Autodesk Inventor part; units mm, degrees
ref_plane "YZ Plane" through (0, 0, 0) normal (1, 0, 0) x (0, 1, 0)
ref_plane "XZ Plane" through (0, 0, 0) normal (0, 1, 0) x (-1, 0, 0)
ref_plane "XY Plane" through (0, 0, 0) normal (0, 0, 1) x (1, 0, 0)
sketch "Sketch1" plane through (0, 0, 0) normal (0, 0, 1) x (1, 0, 0)
  circle A0 centre (0, 0) radius 11
  dimension "d0" = 22
extrude "Extrusion1" add sketch "Sketch1" along normal mid plane 6
sketch "Sketch3" plane through (0, 0, 3) normal (0, 0, 1) x (1, 0, 0)
  point P0 (0, 0)
hole "Hole1" at (0, 0, 3) direction (0, 0, -1) diameter 10.376 end through all
sketch "Sketch2" plane through (0, 0, 3) normal (0, 0, 1) x (1, 0, 0)
  line L0 (11, 1) -> (10, 1)
  line L1 (10, 1) -> (10, -1)
  line L2 (10, -1) -> (11, -1)
  line L3 (11, -1) -> (11, 1)
  circle A0 centre (0, 0) radius 11 construction
  point P0 (10, 0)
  dimension "d3" = 2
  dimension "d4" = 1
extrude "Extrusion2" cut sketch "Sketch2" against normal through all
pattern_circular "Circular Pattern1" count 4 over 360 about axis through (0, 0, 0) along (0, 0, 1) of "Extrusion2"
chamfer "Chamfer1" distance 1 angle 45 4 edges at (7.7782, -7.7782, 3) (7.7782, 7.7782, 3) (-7.7782, 7.7782, 3) (-7.7782, -7.7782, 3)
properties material "Stainless Steel"
Read the model definition and answer for the solid it produces. Units are mm, in the model's axes. A direction names the side the tool comes from. Give positions to 0.01 mm unless a question says otherwise; leave off trailing zeros. Loops run counter-clockwise (first coordinate to the right, second up) from the corner with the lowest first, then second, coordinate; pieces in that order, holes last.
Item 1: For faces 1 (the flat face through (1, -10.5, 0)), 2 (the flat face through (-10.5, 1, 0)), 3 (the flat face through (0, 10, 0)), 4 (the flat face through (10.5, 1, 0)), determine the directions among +Z, -Z, +X, -X, +Y, -Y from which every point of the face is accessible in a straight line to the end or side of a thin tool.
Item 2: Each of these flat-tipped pins is pushed along its axis until it touches: pin 1 Ø1 at (x, z) = (2, 0) entering from +Y; pin 2 Ø1.6 at (x, z) = (0, 0.5) entering from +Y; pin 3 Ø0.8 at (x, z) = (10.5, 0) entering from -Y. Where does it stop, or does it pass through?
Item 3: Find the intervals of material crossed by line 1 along Y through (x, z) = (0, 0.8); line 2 along Y through (x, z) = (-0.75, 0.25), in increasing order.
Item 4: The mould has two halves that part along Y. Classify faces 5 (the flat face through (5, -2, -3)), 6 (the conical face through (-7.116, -7.272, 2.826)), 7 (the flat face through (10, 0, 0)): released by +Y, released by -Y, zero draft, split by the parting line, or undercut.
Item 5: The part is cut by section A-A (z = 1). Write down the section's boundary in (x, y), and give its area (3 significant figures).
Taken from the geometry:
1. face 1: +Z, -Z, -Y
1. face 2: +Z, -Z, -X
1. face 3: +Z, -Z, +Y
1. face 4: +Z, -Z, +X
2. pin 1: stops at y = 10.9
2. pin 2: stops at y = 10
2. pin 3: stops at y = -4.36
3. line 1: y = -10 to -5.19, 5.19 to 10
3. line 2: y = -10 to -5.13, 5.13 to 10
4. face 5: zero draft
4. face 6: released by -Y
4. face 7: undercut
5. outline: (-10.95, -1) arc R11 ccw to (-1, -10.95) - (-1, -10) - (1, -10) - (1, -10.95) arc R11 ccw to (10.95, -1) - (10, -1) - (10, 1) - (10.95, 1) arc R11 ccw to (1, 10.95) - (1, 10) - (-1, 10) - (-1, 10.95) arc R11 ccw to (-10.95, 1) - (-10, 1) - (-10, -1) - close; hole circle Ø10.38 at (0, 0)
5. area: 288 mm2
